Autodesk Fusion 360 part; units mm, degrees
sketch "Sketch1" plane through (0, 0, 0) normal (0, 0, 1) x (1, 0, 0)
  circle A0 centre (0, 0) radius 7
  circle A1 centre (0, 0) radius 22.5
  circle A2 centre (0, 0) radius 38
  dimension "d1" = 45
  dimension "d2" = 14
  dimension "d3" = 76
extrude "Extrude1" add sketch "Sketch1" along normal blind 20 contours A1
sketch "Sketch2" plane through (0, 0, 0) normal (0, 0, 1) x (1, 0, 0)
  circle A0 centre (0.2654, -30.1553) radius 2.5
  dimension "d8" = 5
extrude "Extrude4" add sketch "Sketch1" along normal blind 20 contours A1 | A2
extrude "Extrude5" cut sketch "Sketch2" along normal blind 6.312
pattern_circular "C-Pattern2" count 3 over 360 about axis through (0, 0, 20) along (0, 0, 1) of "Extrude5"
For this review, take the finished solid that the model builds, in its own axes (mm). A direction names the side the tool comes from. Round coordinates to 2 decimals unless told otherwise and drop trailing zeros. Write each loop counter-clockwise with the first axis right and the second up, starting at its lowest first coordinate (ties: lowest second). Pieces come first, ordered by that corner, then holes.
1) For line 1 along X through (y, z) = (-6, 6.75); line 2 along X through (y, z) = (-1.5, 13.5); line 3 along Y through (x, z) = (22.5, 14), list the stretches that pass through material, from the lowest coordinate up.
Answer below:
line 1: x = -37.52 to -3.61, 3.61 to 37.52
line 2: x = -37.97 to -6.84, 6.84 to 37.97
line 3: y = -30.62 to 30.62
2) Take a section at C-C on z = 9.25. Give the boundary of the cut face in (x, y), then the cut area to 3 significant figures.
Answer below:
outline: circle Ø76 at (0, 0); hole circle Ø14 at (0, 0)
area: 4,380 mm2
3) Mouldability with a two-part tool opening along Y and no side actions: class faces 3 (the face through (6.466, 2.681, 9.86)), 4 (the face through (-1, -8, 0)), 5 (the face through (17.535, 33.713, 9.86)) as +Y half, -Y half, draft (parallel to the pull), parting line (faces both ways), or undercut.
Answer below:
face 3: undercut
face 4: draft
face 5: parting line
4) Take a section at A-A on y = 0. Give the boundary of the cut face in (x, z).
Answer below:
outline: (-38, 0) - (-7, 0) - (-7, 20) - (-38, 20) - close; (7, 0) - (38, 0) - (38, 20) - (7, 20) - close
5) Take a section at B-B on x = 0. Give the boundary of the cut face in (y, z), then the cut area to 3 significant figures.
Answer below:
outline: (-38, 0) - (-32.64, 0) - (-32.64, 6.31) - (-27.67, 6.31) - (-27.67, 0) - (-7, 0) - (-7, 20) - (-38, 20) - close; (7, 0) - (38, 0) - (38, 20) - (7, 20) - close
area: 1,210 mm2
6) Insertion check: pin 1 Ø5 at (x, z) = (16, 12.5) entering from -Y; pin 2 Ø16 at (x, y) = (0, 0) entering from -Z; pin 3 Ø1.5 at (x, y) = (1.5, -30.5) entering from -Z; pin 4 Ø6 at (x, z) = (0.5, 3) entering from +Y. Each pin has a flat end and moves straight along its axis. Give the tip position at first contact, or say it passes through.
Answer below:
pin 1: stops at y = -35.52
pin 2: stops at z = 0
pin 3: stops at z = 6.31
pin 4: stops at y = 38
7) Machinability: for faces 1 (the face through (-23.863, 14.097, 3.112)), 2 (the face through (-1, -8, 20)), which of the approach directions +Z, -Z, +X, -X, +Y, -Y give a long, thin tool a straight path to every point of the face, cutting with its end or side? Answer none if there is none.
Answer below:
face 1: -Z
face 2: +Z, +X, -X, +Y, -Y
8) Take a section at D-D on x = 26. Give the boundary of the cut face in (y, z).
Answer below:
outline: (-27.71, 0) - (12.81, 0) - (12.81, 6.31) - (17.81, 6.31) - (17.81, 0) - (27.71, 0) - (27.71, 20) - (-27.71, 20) - close
